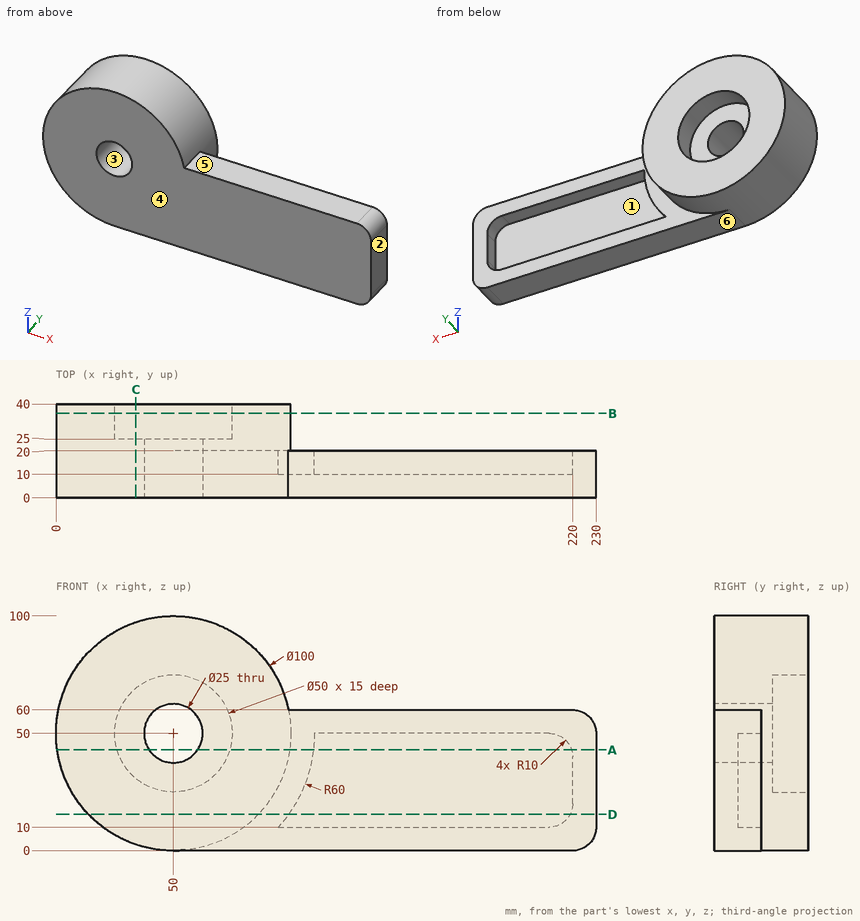
The drawing under review shows one solid part. Ordinate dimensions are in mm from its lowest x, y, z. A direction names the side the tool comes from. Round coordinates to 2 decimals unless told otherwise and drop trailing zeros. Write each loop counter-clockwise with the first axis right and the second up, starting at its lowest first coordinate (ties: lowest second). Pieces come first, ordered by that corner, then holes. Notation, with made-up numbers: (15.5, -30.75) - (66.5, -30.75) arc R9 cw to (66.5, -20.75) - close; hole circle Ø9 at (67, 70.5). An arc over 180 degrees is marked (long way). One line per question, with ' | ' between items.
Item 1: To check wall thickness, follow probe 1 along Z at (x, y) = (50, 30.5); probe 2 along Z at (x, y) = (50, 8.25); probe 3 along Y at (x, z) = (182.5, 58). State the ranges of each line that lie inside material, in increasing order.
Resolved:
probe 1: z = 0 to 25, 75 to 100 | probe 2: z = 0 to 37.5, 62.5 to 100 | probe 3: y = 0 to 20
Item 2: For P1, Ø3, axis at y = 16, z = 33.5, coming from the -X side; P2, Ø1.5, axis at x = 31.5, z = 44.5, coming from the -Y side; P3, Ø20, axis at x = 179.5, z = 38.5, coming from the +Y side; P4, Ø10, axis at x = 132, y = 12, coming from the +Z side, all flat-tipped, find the tip position at first contact; note any pin that passes through.
Resolved:
P1: stops at x = 2.3 | P2: stops at y = 0 | P3: stops at y = 10 | P4: stops at z = 60
Item 3: The part is to be moulded in two halves that separate along Z. For the marked faces 3, 4, 5 and 6, say which applies: pulls with the +Z half, pulls with the -Z half, needs draft (parallel to the pull), parting line crosses it, or undercut.
Resolved:
face 3: undercut | face 4: needs draft | face 5: pulls with the +Z half | face 6: pulls with the -Z half
Item 4: Add section C-C, the plane x = 34. Give the boundary of the cut face in (y, z), then the cut area to 3 significant figures.
Resolved:
outline: (0, 2.63) - (40, 2.63) - (40, 30.79) - (25, 30.79) - (25, 69.21) - (40, 69.21) - (40, 97.37) - (0, 97.37) - close | area: 3,210 mm2
Item 5: Add section A-A, the plane z = 43. Give the boundary of the cut face in (x, y).
Resolved:
outline: (0.49, 0) - (39.64, 0) - (39.64, 25) - (26, 25) - (26, 40) - (0.49, 40) - close; (60.36, 0) - (230, 0) - (230, 20) - (219.54, 20) - (219.54, 10) - (109.59, 10) - (109.59, 20) - (99.51, 20) - (99.51, 40) - (74, 40) - (74, 25) - (60.36, 25) - close
Item 6: Add section B-B, the plane y = 36. Give the boundary of the cut face in (x, z).
Resolved:
outline: circle Ø100 at (50, 50); hole circle Ø50 at (50, 50)
Item 7: Add section D-D, the plane z = 15.5. Give the boundary of the cut face in (x, y), then the cut area to 3 significant figures.
Resolved:
outline: (13.81, 0) - (230, 0) - (230, 20) - (218.93, 20) - (218.93, 10) - (99.09, 10) - (99.09, 20) - (86.19, 20) - (86.19, 40) - (13.81, 40) - close | area: 4,570 mm2
Item 8: For the marked faces 1 and 2, list the 3-axis set-ups (+Z, -Z, +X, -X, +Y, -Y) from which the entire face can be reached by the end or side of a thin tool; tool diameter is ignored.
Resolved:
face 1: +Y | face 2: +Z, -Z, +X, +Y, -Y
